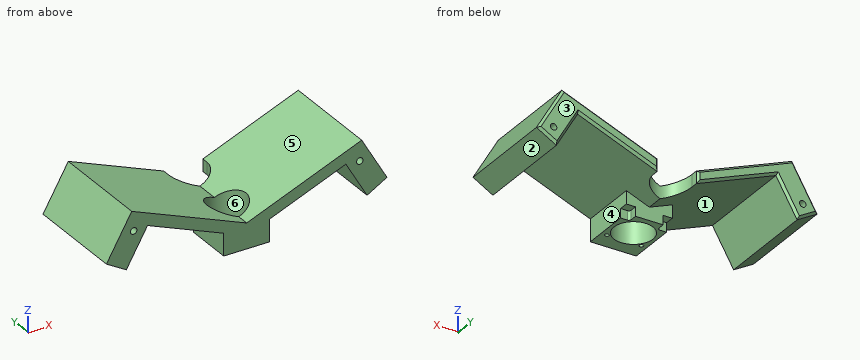
Autodesk Inventor part; units mm, degrees
ref_plane "Work Plane1" through (0, 0, 0) normal (0, 0, -1) x (0, 1, 0)
ref_plane "XZ Plane" through (0, 0, 0) normal (0, 1, 0) x (-1, 0, 0)
ref_plane "XY Plane" through (0, 0, 0) normal (0, 0, 1) x (1, 0, 0)
sketch "Sketch1" plane through (0, 0, 0) normal (0, 1, 0) x (-1, 0, 0)
  line L0 (-56.669873, -1.552559) -> (-61, 0.947441)
  line L1 (56.669873, -1.552559) -> (61, 0.947441)
  line L2 (61, 0.947441) -> (50, 20)
  line L3 (-50, 20) -> (-61, 0.947441)
  line L4 (0, 0) -> (-50, 20)
  line L5 (0, 0) -> (50, 20)
  line L6 (-50, 20) -> (-55, 11.339746)
  line L7 (50, 20) -> (55, 11.339746)
  line L8 (-56.669873, -1.552559) -> (-52.339746, -4.052559)
  line L9 (56.669873, -1.552559) -> (52.339746, -4.052559)
  line L10 (50, 20) -> (52.5, 15.669873)
  line L11 (-50, 20) -> (-52.5, 15.669873)
  line L12 (-43.119361, 11.917617) -> (0, -5.330127)
  line L13 (43.119361, 11.917617) -> (0, -5.330127)
  line L14 (-52.339746, -4.052559) -> (-43.119361, 11.917617)
  line L15 (43.119361, 11.917617) -> (52.339746, -4.052559)
  dimension "d1" = 5
  dimension "d2" = 5
  dimension "d3" = 5
  dimension "d4" = 5
extrude "Extrusion1" add sketch "Sketch1" along normal blind 45
sketch "Sketch2" plane through (0, 0, 0) normal (0, -1, 0) x (1, 0, 0)
  line L0 (61, 0.947441) -> (52.339746, -4.052559)
  line L1 (50, 20) -> (61, 0.947441)
  line L2 (0, 0) -> (50, 20)
  line L3 (-50, 20) -> (0, 0)
  line L4 (-61, 0.947441) -> (-50, 20)
  line L5 (-52.339746, -4.052559) -> (-61, 0.947441)
  line L6 (-43.119361, 11.917617) -> (-52.339746, -4.052559)
  line L7 (0, -5.330127) -> (-43.119361, 11.917617)
  line L8 (43.119361, 11.917617) -> (0, -5.330127)
  line L9 (52.339746, -4.052559) -> (43.119361, 11.917617)
  line L10 (-56.669873, -1.552559) -> (-49.169873, 11.437822)
  line L11 (56.669873, -1.552559) -> (49.169873, 11.437822)
  circle A0 centre (49.169873, 11.437822) radius 1.4
  circle A1 centre (-49.169873, 11.437822) radius 1.4
  dimension "d8" = 15
  dimension "d9" = 15
  dimension "d10" = 2.8
  dimension "d11" = 2.8
extrude "Extrusion2" cut sketch "Sketch2" against normal blind 30 contours A0 | A1
sketch "Sketch3" plane through (0, 45, 0) normal (0, 1, 0) x (1, 0, 0)
  circle A0 centre (-54.169873, -2.777568) radius 1.4
  circle A1 centre (54.169873, -2.777568) radius 1.4
  line L0 (61, -0.947441) -> (52.339746, 4.052559)
  line L1 (52.339746, 4.052559) -> (43.119361, -11.917617)
  line L2 (43.119361, -11.917617) -> (0, 5.330127)
  line L3 (0, 5.330127) -> (-43.119361, -11.917617)
  line L4 (-43.119361, -11.917617) -> (-52.339746, 4.052559)
  line L5 (-52.339746, 4.052559) -> (-61, -0.947441)
  line L6 (-61, -0.947441) -> (-50, -20)
  line L7 (-50, -20) -> (0, 0)
  line L8 (0, 0) -> (50, -20)
  line L9 (50, -20) -> (61, -0.947441)
  dimension "d30" = 2.8
  dimension "d31" = 2.8
extrude "Extrusion3" cut sketch "Sketch3" against normal blind 20 contours A0 | A1
chamfer "Chamfer1" distance 1 angle 45 2 edges at (-56.6699, 45, -1.5526) (56.6699, 45, -1.5526)
chamfer "Chamfer2" distance 1 angle 45 8 edges at (55.25, 45, 10.9067) (47.4796, 45, 4.3655) (21.5597, 45, 3.2937) (-21.5597, 45, 3.2937) (-47.4796, 45, 4.3655) (-55.25, 45, 10.9067) (-25, 45, 10) (25, 45, 10)
ref_plane "Work Plane1" through (0, 0, 0) normal (0, 0, -1) x (0, 1, 0)
sketch "Sketch4" plane through (0, 0, 0) normal (0, 0, -1) x (0, 1, 0)
  line L0 (0, 0) -> (0, -10)
  line L1 (0, 0) -> (0, -43.119361)
  line L2 (0, -10) -> (25, -10)
  line L3 (25, -10) -> (25, 10)
  line L4 (25, 10) -> (0, 10)
  line L5 (0, 10) -> (0, 0)
  dimension "d33" = 10
  dimension "d34" = 25
  dimension "d35" = 20
extrude "Extrusion4" add sketch "Sketch4" along normal blind 11
sketch "Sketch5" plane through (0, 0, -11) normal (0, 0, -1) x (-1, 0, 0)
  circle A0 centre (0, 14) radius 8.5
  circle A1 centre (-7.5, 7.5) radius 0.9
  circle A2 centre (7.5, 7.5) radius 0.9
  line L0 (0, 14) -> (0, 41)
  line L1 (0, 0) -> (0, 44)
  line L2 (-8.5, 41) -> (-8.5, 45)
  line L3 (0, 45) -> (-43.552262, 45)
  line L4 (8.5, 41) -> (8.5, 45)
  line L5 (0, 45) -> (49.567099, 45)
  line L6 (8.5, 45) -> (-8.5, 45)
  arc A3 (-8.5, 41) -> (8.5, 41) centre (0, 41) ccw
  dimension "d38" = 17
  dimension "d39" = 1.8
  dimension "d40" = 1.8
  dimension "d41" = 27
extrude "Extrusion5" cut sketch "Sketch5" against normal through all contours A0 L1 L0 | L0 L1 A0 | L2 L3 L5 L4 A3
chamfer "Chamfer3" distance 1 angle 45 2 edges at (8.5, 45, 0.7349) (-8.5, 45, 0.7349)
sketch "Sketch6" plane through (0, 0, -11) normal (0, 0, -1) x (-1, 0, 0)
  circle A0 centre (-7.5, 7.5) radius 0.9
  circle A1 centre (7.5, 7.5) radius 0.9
  point P0 (0, 0)
  point P1 (0, 0)
  dimension "d49" = 1.8
  dimension "d50" = 1.8
extrude "Extrusion6" cut sketch "Sketch6" against normal blind 10
sketch "Sketch7" plane through (0, 0, -11) normal (0, 0, -1) x (-1, 0, 0)
  line L0 (-10, 25) -> (10, 25)
  line L1 (-10, 25) -> (-6, 25)
  line L2 (-6, 25) -> (-6, 21)
  line L3 (-6, 21) -> (-10, 21)
  line L4 (10, 25) -> (6, 25)
  line L5 (-10, 25) -> (10, 25)
  line L6 (6, 25) -> (6, 21)
  line L7 (6, 21) -> (10, 21)
  line L8 (10, 25) -> (10, 21)
  line L9 (-10, 25) -> (-6, 25)
  line L10 (-6, 25) -> (-6, 21)
  line L11 (-6, 21) -> (-10, 21)
  line L12 (-10, 21) -> (-10, 25)
  line L13 (6, 25) -> (10, 25)
  line L14 (10, 25) -> (10, 21)
  line L15 (10, 21) -> (6, 21)
  line L16 (6, 21) -> (6, 25)
  dimension "d54" = 4
  dimension "d55" = 4
  dimension "d56" = 4
extrude "Extrusion7" cut sketch "Sketch7" against normal blind 4
fillet "Fillet1" radius 1 2 edges at (6, 21, -9) (-6, 21, -9)
properties part number "Front Support" material "ABS Plastic"
Can you work these out from the model? Positions are in its coordinate system, mm. Face numbers are marked on the shaded views. A direction names the side the tool comes from. Give positions to 0.01 mm unless a question says otherwise; leave off trailing zeros. Order: outer loops, then holes, each group sorted by start corner. A loop starts at its lowest first (then second) coordinate and runs counter-clockwise, first axis right, second up. Notation, with made-up numbers: M -7.75,37.25 L 43.25,37.25 A27 cw 43.25,63.25 Z; hole C 82,-36 d7. An arc over 180 degrees is marked long. Use one line per item in the form item = value.
Item 1: If we section it at D-D, the plane x = -23.5: Write out the boundary of the cut face in (y, z).
Values follow:
outline = M 0,4.07 L 44,4.07 L 45,5.15 L 45,8.32 L 44,9.4 L 0,9.4 Z
Item 2: If we section it at B-B, the plane z = 7: Write out the boundary of the cut face in (x, y), and give its area (3 significant figures).
Values follow:
outline = M -57.51,0 L -45.96,0 L -45.96,44 L -47.11,45 L -56.35,45 L -57.51,44 Z; M -30.83,0 L -17.5,0 L -17.5,44 L -20.19,45 L -28.13,45 L -30.83,44 Z; M 17.5,0 L 30.83,0 L 30.83,44 L 28.13,45 L 20.19,45 L 17.5,44 Z; M 45.96,0 L 57.51,0 L 57.51,44 L 56.35,45 L 47.11,45 L 45.96,44 Z
area = 2,230 mm^2
Item 3: If we section it at C-C, the plane y = 14: Write out the boundary of the cut face in (x, z), and give its area (3 significant figures).
Values follow:
outline = M -61,0.95 L -52.34,-4.05 L -43.12,11.92 L -10,-1.33 L -10,-11 L -8.5,-11 L -8.5,3.4 L -50,20 Z; M 8.5,-11 L 10,-11 L 10,-1.33 L 43.12,11.92 L 52.34,-4.05 L 61,0.95 L 50,20 L 8.5,3.4 Z; hole C -49.17,11.44 d2.8; hole C 49.17,11.44 d2.8
area = 826 mm^2
Item 4: For the marked faces 4, 5 and 6, which set-ups out of +Z, -Z, +X, -X, +Y, -Y let a thin tool reach every point of the face, with its end or its side?
Values follow:
face_4 = -Z, +Y, -Y
face_5 = +Z, +Y, -Y
face_6 = +Z, -Z
Item 5: Will these pins go through, and if not, where does the flat tip stop? pin 1 Ø4 at (y, z) = (13, 0) entering from -X; pin 2 Ø2 at (x, y) = (-8, 7.5) entering from -Z; pin 3 Ø10 at (x, y) = (0, 14) entering from +Z; pin 4 Ø4 at (y, z) = (39.5, 4.5) entering from -X.
Values follow:
pin_1 = -61
pin_2 = -11
pin_3 = through
pin_4 = -60.1
Item 6: If we section it at A-A, the plane y = 38: Write out the boundary of the cut face in (x, z).
Values follow:
outline = M -61,0.95 L -52.34,-4.05 L -43.12,11.92 L -7.95,-2.15 L -7.95,3.18 L -50,20 Z; M 7.95,-2.15 L 43.12,11.92 L 52.34,-4.05 L 61,0.95 L 50,20 L 7.95,3.18 Z; hole C -54.17,2.78 d2.8; hole C 54.17,2.78 d2.8
Item 7: If I drill on line 1 along Y through (x, z) = (0, -7.75); line 2 along Y through (x, z) = (-7, -8); line 3 along Y through (x, z) = (-7, -6), over which ranges is the centre line in solid material (lowest first)? Write a range as [from, to].
Values follow:
line_1 = [0, 5.5], [22.5, 25]
line_2 = [0, 6.75], [8.25, 9.18], [18.82, 21]
line_3 = [0, 6.75], [8.25, 9.18], [18.82, 25]
Item 8: Thinking about a two-plate mould opening in X: for the marked faces 1, 2 and 3, which applies, pulls with the +X half, pulls with the -X half, needs draft (parallel to the pull), parting line crosses it, or undercut?
Values follow:
face_1 = undercut
face_2 = pulls with the +X half
face_3 = needs draft
